The drawing under review shows one solid part. Ordinate dimensions are in mm from its lowest x, y, z. Coordinates: 2 decimals unless noted, no trailing zeros. Write each loop counter-clockwise with the first axis right and the second up, starting at its lowest first coordinate (ties: lowest second). Pieces come first, ordered by that corner, then holes.
1) For P1, Ø1.2, axis at y = 5, z = 2, coming from the -X side, flat-tipped, find the tip position at first contact; note if it passes through.
2) Add section C-C, the plane x = 6.5. State the section outline as (y, z) points.
3) Add section A-A, the plane y = 2.75. State the section outline as (x, z) points.
4) Add section B-B, the plane z = 6.75. State the section outline as (x, y) points.
5) For line 1 (X direction, y = 2.4, z = 4.5); line 2 (Y direction, x = 4.75, z = 3.25), list the stretches that pass through material, from the lowest coordinate up.
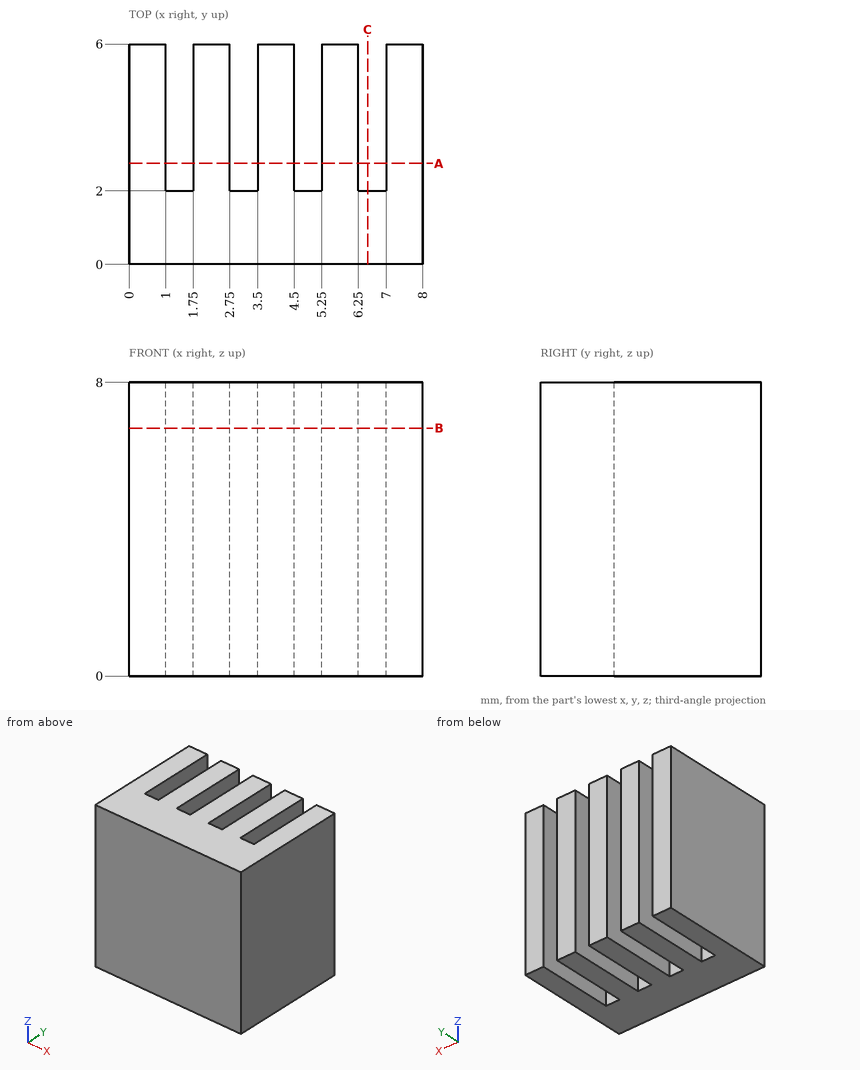
Geometry results:
1. P1: stops at x = 0
2. outline: (0, 0) - (2, 0) - (2, 8) - (0, 8) - close
3. outline: (0, 0) - (1, 0) - (1, 8) - (0, 8) - close; (1.75, 0) - (2.75, 0) - (2.75, 8) - (1.75, 8) - close; (3.5, 0) - (4.5, 0) - (4.5, 8) - (3.5, 8) - close; (5.25, 0) - (6.25, 0) - (6.25, 8) - (5.25, 8) - close; (7, 0) - (8, 0) - (8, 8) - (7, 8) - close
4. outline: (0, 0) - (8, 0) - (8, 6) - (7, 6) - (7, 2) - (6.25, 2) - (6.25, 6) - (5.25, 6) - (5.25, 2) - (4.5, 2) - (4.5, 6) - (3.5, 6) - (3.5, 2) - (2.75, 2) - (2.75, 6) - (1.75, 6) - (1.75, 2) - (1, 2) - (1, 6) - (0, 6) - close
5. line 1: x = 0 to 1, 1.75 to 2.75, 3.5 to 4.5, 5.25 to 6.25, 7 to 8
5. line 2: y = 0 to 2
